from build123d import *

# Parameters (mm, degrees)
SKETCH_R     = 1.5
SKETCH_R_2   = 2.5
PAD_DEPTH    = 3.5
CHAMFER_SIZE = 2


with BuildPart() as part:
    # Sketch → Pad (new body)
    with BuildSketch(Plane.XY):
        Polygon((-44, 69), (44, 69), (49, 64), (49, -64), (44, -69), (-44, -69), (-49, -64), (-49, 64), align=None)
        with Locations((-17.25, 50.25)):
            Circle(SKETCH_R, mode=Mode.SUBTRACT)
        with Locations((34.75, 50.25)):
            Circle(SKETCH_R, mode=Mode.SUBTRACT)
        with Locations((34.75, 25.25)):
            Circle(SKETCH_R, mode=Mode.SUBTRACT)
        with Locations((-17.25, 25.25)):
            Circle(SKETCH_R, mode=Mode.SUBTRACT)
        with Locations((-34.75, -43)):
            Circle(SKETCH_R, mode=Mode.SUBTRACT)
        with Locations((-34.75, 6.5)):
            Circle(SKETCH_R, mode=Mode.SUBTRACT)
        with Locations((34.75, 6.5)):
            Circle(SKETCH_R, mode=Mode.SUBTRACT)
        with Locations((34.75, -43)):
            Circle(SKETCH_R, mode=Mode.SUBTRACT)
        with Locations((-44, 0)):
            Circle(SKETCH_R_2, mode=Mode.SUBTRACT)
        with Locations((0, 64)):
            Circle(SKETCH_R_2, mode=Mode.SUBTRACT)
        with Locations((44, 0)):
            Circle(SKETCH_R_2, mode=Mode.SUBTRACT)
        with Locations((0, -64)):
            Circle(SKETCH_R_2, mode=Mode.SUBTRACT)
        with BuildLine():
            ThreePointArc((-28.5, -49), (-30, -47.5), (-31.5, -49))
            Line((-31.5, -49), (-31.5, -54))
            ThreePointArc((-31.5, -54), (-30, -55.5), (-28.5, -54))
            Line((-28.5, -54), (-28.5, -49))
        make_face(mode=Mode.SUBTRACT)
        with BuildLine():
            ThreePointArc((-13.5, -49), (-15, -47.5), (-16.5, -49))
            Line((-16.5, -49), (-16.5, -54))
            ThreePointArc((-16.5, -54), (-15, -55.5), (-13.5, -54))
            Line((-13.5, -54), (-13.5, -49))
        make_face(mode=Mode.SUBTRACT)
        with BuildLine():
            ThreePointArc((1.5, -49), (0, -47.5), (-1.5, -49))
            Line((-1.5, -49), (-1.5, -54))
            ThreePointArc((-1.5, -54), (0, -55.5), (1.5, -54))
            Line((1.5, -54), (1.5, -49))
        make_face(mode=Mode.SUBTRACT)
        with BuildLine():
            ThreePointArc((16.5, -49), (15, -47.5), (13.5, -49))
            Line((13.5, -49), (13.5, -54))
            ThreePointArc((13.5, -54), (15, -55.5), (16.5, -54))
            Line((16.5, -54), (16.5, -49))
        make_face(mode=Mode.SUBTRACT)
        with BuildLine():
            ThreePointArc((31.5, -49), (30, -47.5), (28.5, -49))
            Line((28.5, -49), (28.5, -54))
            ThreePointArc((28.5, -54), (30, -55.5), (31.5, -54))
            Line((31.5, -54), (31.5, -49))
        make_face(mode=Mode.SUBTRACT)
        with BuildLine():
            ThreePointArc((-34.25, 44.25), (-35.75, 42.75), (-34.25, 41.25))
            Line((-34.25, 41.25), (-29.25, 41.25))
            ThreePointArc((-29.25, 41.25), (-27.75, 42.75), (-29.25, 44.25))
            Line((-29.25, 44.25), (-34.25, 44.25))
        make_face(mode=Mode.SUBTRACT)
        with BuildLine():
            ThreePointArc((-34.25, 34.25), (-35.75, 32.75), (-34.25, 31.25))
            Line((-34.25, 31.25), (-29.25, 31.25))
            ThreePointArc((-29.25, 31.25), (-27.75, 32.75), (-29.25, 34.25))
            Line((-29.25, 34.25), (-34.25, 34.25))
        make_face(mode=Mode.SUBTRACT)
        with BuildLine():
            ThreePointArc((-43.25, 23.5), (-44.75, 25), (-46.25, 23.5))
            Line((-46.25, 23.5), (-46.25, 18.5))
            ThreePointArc((-46.25, 18.5), (-44.75, 17), (-43.25, 18.5))
            Line((-43.25, 18.5), (-43.25, 23.5))
        make_face(mode=Mode.SUBTRACT)
        with BuildLine():
            ThreePointArc((-33.25, 23.5), (-34.75, 25), (-36.25, 23.5))
            Line((-36.25, 23.5), (-36.25, 18.5))
            ThreePointArc((-36.25, 18.5), (-34.75, 17), (-33.25, 18.5))
            Line((-33.25, 18.5), (-33.25, 23.5))
        make_face(mode=Mode.SUBTRACT)
    extrude(amount=PAD_DEPTH)

    # Chamfer
    chamfer_edges = [part.edges().sort_by_distance(p)[0] for p in [
        (41.5, 0, 3.5),
        (-2.5, -64, 3.5),
        (-46.5, 0, 3.5),
        (-2.5, 64, 3.5),
    ]]
    chamfer(chamfer_edges, length=CHAMFER_SIZE)


solid = part.part
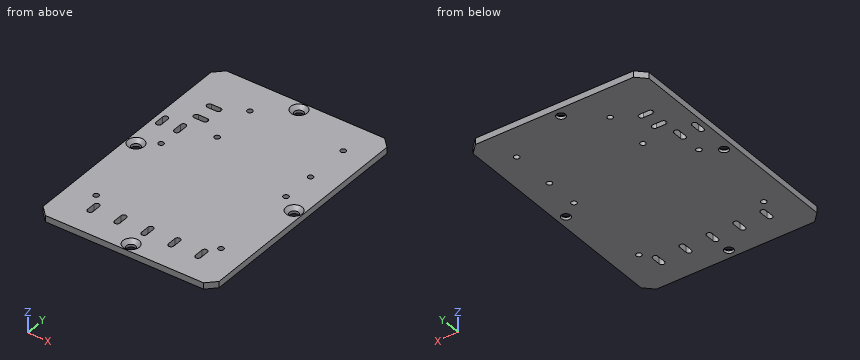
Part model, mm, in its own coordinate system. Give positions to 0.01 mm unless a question says otherwise; leave off trailing zeros. Write each loop counter-clockwise with the first axis right and the second up, starting at its lowest first coordinate (ties: lowest second). Pieces come first, ordered by that corner, then holes.
1) Probe L1, parallel to X at y = 19, z = 0.3; L2, parallel to Y at x = 34.75, z = 0.9; L3, parallel to X at y = -51.5, z = 0.55. List the from-to ranges inside material, lowest first.
Resolved:
L1: x = -49 to -46.25, -43.25 to -36.25, -33.25 to 49
L2: y = -69 to -44.5, -41.5 to 5, 8 to 23.75, 26.75 to 48.75, 51.75 to 69
L3: x = -49 to -31.5, -28.5 to -16.5, -13.5 to -1.5, 1.5 to 13.5, 16.5 to 28.5, 31.5 to 49
2) Pin check, flat tip, straight feed: pin 1 (8 mm diameter, centred on x = 0, y = -64, fed in from -Z). Stop position of the tip, or through.
Resolved:
pin 1: stops at z = 0
3) Cut at A-A on y = 42.75. Write the cut outline in (x, z).
Resolved:
outline: (-49, 0) - (-35.75, 0) - (-35.75, 3.5) - (-49, 3.5) - close; (-27.75, 0) - (49, 0) - (49, 3.5) - (-27.75, 3.5) - close
4) Cut at B-B on z = 2.2. State how many separate pieces and enclosed holes the cut face has, then the cut area to 3 significant figures.
Resolved:
separate pieces: 1
enclosed holes: 21
area: 13,100 mm2
